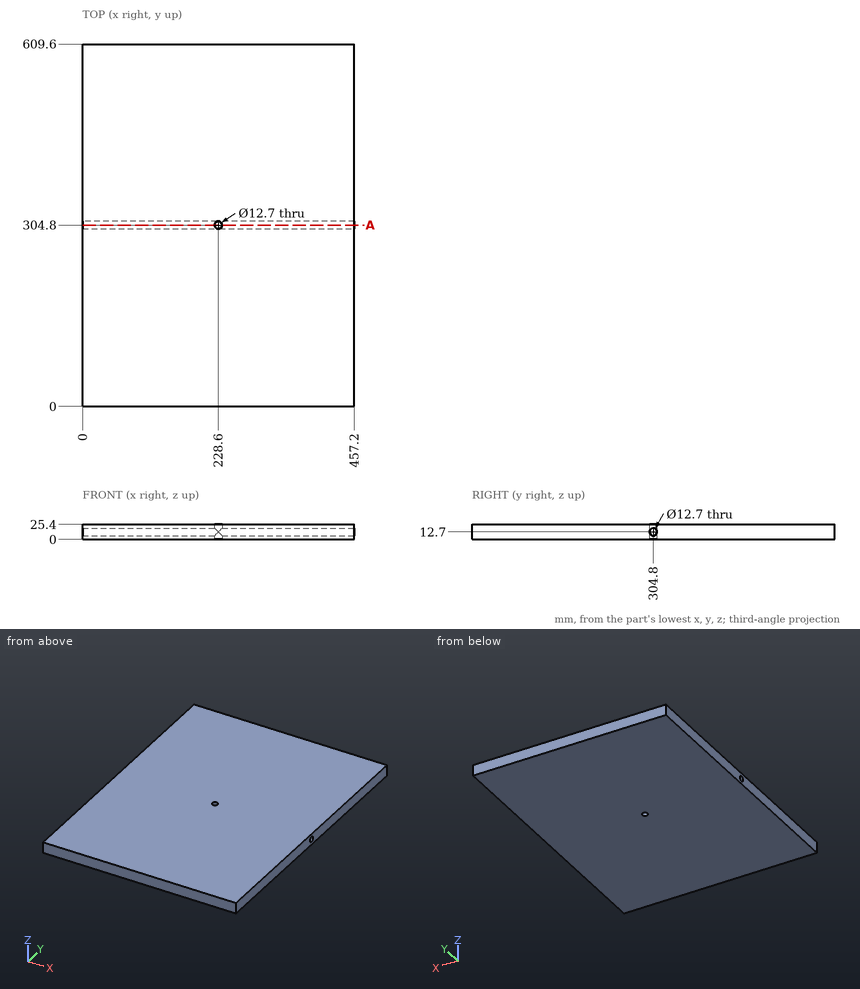
Source: three-view drawing plus pictorial views. Frame: mm from the lowest corner of the part. Round coordinates to 2 decimals unless told otherwise and drop trailing zeros. Order: outer loops, then holes, each group sorted by start corner. A loop starts at its lowest first (then second) coordinate and runs counter-clockwise, first axis right, second up. Notation, with made-up numbers: (14, -30) - (30, -30) arc R6 ccw to (30, -20) - close; hole circle Ø8 at (32, 79). An arc over 180 degrees is marked (long way). Use a Markdown table: item, result.
1. Material intervals for probe 1 along Y at (x, z) = (172.5, 12.7); probe 2 along Z at (x, y) = (107, 304); probe 3 along X at (y, z) = (304.8, 21.25), sorted ascending.
Evaluation:
| item | result |
|---|---|
| probe 1 | 0 to 298.45, 311.15 to 609.6 |
| probe 2 | 0 to 6.4, 19 to 25.4 |
| probe 3 | 0 to 222.25, 234.95 to 457.2 |
2. Section A-A on y = 304.8. Return the cut outline in (x, z), then the cut area to 3 significant figures.
Evaluation:
| item | result |
|---|---|
| outline | (0, 0) - (222.25, 0) - (222.25, 6.35) - (0, 6.35) - close; (0, 19.05) - (222.25, 19.05) - (222.25, 25.4) - (0, 25.4) - close; (234.95, 0) - (457.2, 0) - (457.2, 6.35) - (234.95, 6.35) - close; (234.95, 19.05) - (457.2, 19.05) - (457.2, 25.4) - (234.95, 25.4) - close |
| area | 5,650 mm^2 |
3. First-contact query: pin 1 (20.5 mm diameter, centred on x = 228.6, y = 304.8, fed in from +Z). Flat tip, straight axial feed; report the tip coordinate or a pass-through.
Evaluation:
| item | result |
|---|---|
| pin 1 | z = 25.4 |
